from build123d import *

# Parameters (mm, degrees)
BOSS_EXTRUDE1_DEPTH = 3
SKETCH2_W           = 3
SKETCH2_H           = 41.3
BOSS_EXTRUDE2_DEPTH = 48
CUT_EXTRUDE1_DEPTH  = 48
CHAMFER1_SIZE       = 4


with BuildPart() as part:
    # Sketch1 → Boss-Extrude1 (new body)
    with BuildSketch(Plane(origin=(0, 0, 0), x_dir=(1, 0, 0), z_dir=(0, 1, 0))):
        with BuildLine():
            Line((15.35, 20.65), (-17.5, 20.65))
            Line((-17.5, 20.65), (-17.5, -20.65))
            Line((-17.5, -20.65), (15.35, -20.65))
            ThreePointArc((15.35, -20.65), (16.87027958, -20.02027958), (17.5, -18.5))
            Line((17.5, -18.5), (17.5, -13.25))
            ThreePointArc((17.5, -13.25), (16.87027958, -11.72972042), (15.35, -11.1))
            Line((15.35, -11.1), (6.65, -11.1))
            ThreePointArc((6.65, -11.1), (5.12972042, -10.47027958), (4.5, -8.95))
            Line((4.5, -8.95), (4.5, -4.3))
            ThreePointArc((4.5, -4.3), (3.87027958, -2.77972042), (2.35, -2.15))
            Line((2.35, -2.15), (1.5, -2.15))
            ThreePointArc((1.5, -2.15), (-0.65, 0), (1.5, 2.15))
            Line((1.5, 2.15), (2.35, 2.15))
            ThreePointArc((2.35, 2.15), (3.87027958, 2.77972042), (4.5, 4.3))
            Line((4.5, 4.3), (4.5, 8.95))
            ThreePointArc((4.5, 8.95), (5.12972042, 10.47027958), (6.65, 11.1))
            Line((6.65, 11.1), (15.35, 11.1))
            ThreePointArc((15.35, 11.1), (16.87027958, 11.72972042), (17.5, 13.25))
            Line((17.5, 13.25), (17.5, 18.5))
            ThreePointArc((17.5, 18.5), (16.87027958, 20.02027958), (15.35, 20.65))
        make_face()
        with BuildLine():
            Line((-5.85, -12.7), (-5.85, -15.9))
            ThreePointArc((-5.85, -15.9), (-8, -18.05), (-10.15, -15.9))
            Line((-10.15, -15.9), (-10.15, -12.7))
            ThreePointArc((-10.15, -12.7), (-8, -10.55), (-5.85, -12.7))
        make_face(mode=Mode.SUBTRACT)
        with BuildLine():
            Line((-1.7, -8.5), (-4.8, -8.5))
            ThreePointArc((-4.8, -8.5), (-6.95, -6.35), (-4.8, -4.2))
            Line((-4.8, -4.2), (-1.7, -4.2))
            ThreePointArc((-1.7, -4.2), (0.45, -6.35), (-1.7, -8.5))
        make_face(mode=Mode.SUBTRACT)
        with BuildLine():
            Line((3.65, -12.7), (3.65, -15.9))
            ThreePointArc((3.65, -15.9), (1.5, -18.05), (-0.65, -15.9))
            Line((-0.65, -15.9), (-0.65, -12.7))
            ThreePointArc((-0.65, -12.7), (1.5, -10.55), (3.65, -12.7))
        make_face(mode=Mode.SUBTRACT)
        with BuildLine():
            Line((14.2, -18.05), (11, -18.05))
            ThreePointArc((11, -18.05), (8.85, -15.9), (11, -13.75))
            Line((11, -13.75), (14.2, -13.75))
            ThreePointArc((14.2, -13.75), (16.35, -15.9), (14.2, -18.05))
        make_face(mode=Mode.SUBTRACT)
        with BuildLine():
            ThreePointArc((-4.8, 4.2), (-6.95, 6.35), (-4.8, 8.5))
            Line((-4.8, 8.5), (-1.7, 8.5))
            ThreePointArc((-1.7, 8.5), (0.45, 6.35), (-1.7, 4.2))
            Line((-1.7, 4.2), (-4.8, 4.2))
        make_face(mode=Mode.SUBTRACT)
        with BuildLine():
            ThreePointArc((-10.15, 15.9), (-8, 18.05), (-5.85, 15.9))
            Line((-5.85, 15.9), (-5.85, 12.7))
            ThreePointArc((-5.85, 12.7), (-7.123986993, 10.736558834), (-9.436140662, 11.1))
            ThreePointArc((-9.436140662, 11.1), (-9.963441166, 11.823986993), (-10.15, 12.7))
            Line((-10.15, 12.7), (-10.15, 15.9))
        make_face(mode=Mode.SUBTRACT)
        with BuildLine():
            ThreePointArc((-0.65, 15.9), (1.5, 18.05), (3.65, 15.9))
            Line((3.65, 15.9), (3.65, 12.7))
            ThreePointArc((3.65, 12.7), (1.5, 10.55), (-0.65, 12.7))
            Line((-0.65, 12.7), (-0.65, 15.9))
        make_face(mode=Mode.SUBTRACT)
        with BuildLine():
            ThreePointArc((11, 13.75), (8.85, 15.9), (11, 18.05))
            Line((11, 18.05), (14.2, 18.05))
            ThreePointArc((14.2, 18.05), (16.35, 15.9), (14.2, 13.75))
            Line((14.2, 13.75), (11, 13.75))
        make_face(mode=Mode.SUBTRACT)
    extrude(amount=BOSS_EXTRUDE1_DEPTH)

    # Sketch2 → Boss-Extrude2 (add)
    with BuildSketch(Plane(origin=(0, 3, 0), x_dir=(1, 0, 0), z_dir=(0, 1, 0))):
        with Locations((-16, 0)):
            Rectangle(SKETCH2_W, SKETCH2_H)
    extrude(amount=BOSS_EXTRUDE2_DEPTH)

    # Sketch3 → Cut-Extrude1 (cut)
    with BuildSketch(Plane(origin=(-14.5, 0, 0), x_dir=(0, 0, -1), z_dir=(1, 0, 0))):
        with BuildLine():
            Line((-16, 30.4), (-16, 28.4))
            ThreePointArc((-16, 28.4), (0, 12.4), (16, 28.4))
            Line((16, 28.4), (16, 30.4))
            ThreePointArc((16, 30.4), (0, 46.4), (-16, 30.4))
        make_face()
        with BuildLine():
            Line((17.1, 45.9), (17.1, 43.9))
            ThreePointArc((17.1, 43.9), (15.5, 42.3), (13.9, 43.9))
            Line((13.9, 43.9), (13.9, 45.9))
            ThreePointArc((13.9, 45.9), (15.5, 47.5), (17.1, 45.9))
        make_face()
        with BuildLine():
            Line((-17.1, 45.9), (-17.1, 43.9))
            ThreePointArc((-17.1, 43.9), (-15.5, 42.3), (-13.9, 43.9))
            Line((-13.9, 43.9), (-13.9, 45.9))
            ThreePointArc((-13.9, 45.9), (-15.5, 47.5), (-17.1, 45.9))
        make_face()
        with BuildLine():
            Line((17.1, 12.9), (17.1, 14.9))
            ThreePointArc((17.1, 14.9), (15.5, 16.5), (13.9, 14.9))
            Line((13.9, 14.9), (13.9, 12.9))
            ThreePointArc((13.9, 12.9), (15.5, 11.3), (17.1, 12.9))
        make_face()
        with BuildLine():
            Line((-17.1, 12.9), (-17.1, 14.9))
            ThreePointArc((-17.1, 14.9), (-15.5, 16.5), (-13.9, 14.9))
            Line((-13.9, 14.9), (-13.9, 12.9))
            ThreePointArc((-13.9, 12.9), (-15.5, 11.3), (-17.1, 12.9))
        make_face()
    extrude(amount=-CUT_EXTRUDE1_DEPTH, mode=Mode.SUBTRACT)

    # Chamfer1
    chamfer1_edges = [part.edges().sort_by_distance(p)[0] for p in [
        (-16, 51, 20.65),
        (-16, 51, -20.65),
    ]]
    chamfer(chamfer1_edges, length=CHAMFER1_SIZE)


solid = part.part
For this review, take the finished solid that the model builds, in its own axes (mm). A direction names the side the tool comes from. Coordinates: 2 decimals unless noted, no trailing zeros. Loops run counter-clockwise (first coordinate to the right, second up) from the corner with the lowest first, then second, coordinate; pieces in that order, holes last. Notation, with made-up numbers: (46, 68.5) - (69, 68.5) arc R18 ccw to (69, 78.5) - close; hole circle Ø1 at (-13.75, 39). An arc over 180 degrees is marked (long way). Use a Markdown table: item, result. Add a question column.
Item 1: We need section A-A (z = 0). Give the boundary of the cut face in (x, y).
Item 2: Mouldability with a two-part tool opening along X and no side actions: class faces 1 (the face through (0.45, 1.48, -6.4)), 2 (the face through (-7.95, 1.48, 18.05)), 3 (the face through (-16, 45, 13.9)), 4 (the face through (17.5, 1, 16)) as pulls with the +X half, pulls with the -X half, needs draft (parallel to the pull), parting line crosses it, or undercut.
Item 3: For line 1 (Y direction, x = -12.5, z = 7.5); line 2 (X direction, y = 16.5, z = 15); line 3 (Y direction, x = -15, z = -1), list the stretches that pass through material, from the lowest coordinate up.
Item 4: Tool access review of faces 5 (the face through (13, 1, -18.05)), 6 (the face through (16.89, 1.48, -20)), 7 (the face through (16.89, 1.48, 11.75)), 8 (the face through (-16, 14, -17.1)), 9 (the face through (-15, 16, 20.65)): name each direction out of +Z, -Z, +X, -X, +Y, -Y from which nothing blocks a thin tool from reaching the whole face with its end or side.
Item 5: We need section B-B (z = 5.5). Give the boundary of the cut face in (x, y).
Item 6: Insertion check: pin 1 Ø5 at (x, z) = (-10, -1) entering from -Y; pin 2 Ø5 at (y, z) = (39, -12) entering from +X; pin 3 Ø4 at (x, z) = (13.5, -16.5) entering from +Y; pin 4 Ø1.5 at (y, z) = (1, 6.5) entering from +X. Each pin has a flat end and moves straight along its axis. Give the tip position at first contact, or say it passes through.
Results list:
| question | item | result |
|---|---|---|
| 1 | outline | (-17.5, 0) - (-0.65, 0) - (-0.65, 3) - (-14.5, 3) - (-14.5, 12.4) - (-17.5, 12.4) - close; (-17.5, 46.4) - (-14.5, 46.4) - (-14.5, 51) - (-17.5, 51) - close |
| 2 | face 1 | undercut |
| 2 | face 2 | undercut |
| 2 | face 3 | needs draft |
| 2 | face 4 | pulls with the +X half |
| 3 | line 1 | y = 0 to 3 |
| 3 | line 2 | x = -17.5 to -14.5 |
| 3 | line 3 | y = 0 to 12.43, 46.37 to 51 |
| 4 | face 5 | +Y, -Y |
| 4 | face 6 | -Z, +X, +Y, -Y |
| 4 | face 7 | +X, +Y, -Y |
| 4 | face 8 | +X, -X |
| 4 | face 9 | +Z, +X, -X, +Y, -Y |
| 5 | outline | (-17.5, 0) - (-6.77, 0) - (-6.77, 3) - (-14.5, 3) - (-14.5, 13.38) - (-17.5, 13.38) - close; (-17.5, 45.42) - (-14.5, 45.42) - (-14.5, 51) - (-17.5, 51) - close; (0.27, 0) - (4.5, 0) - (4.5, 3) - (0.27, 3) - close |
| 6 | pin 1 | stops at y = 0 |
| 6 | pin 2 | stops at x = -14.5 |
| 6 | pin 3 | stops at y = 3 |
| 6 | pin 4 | stops at x = 4.5 |
